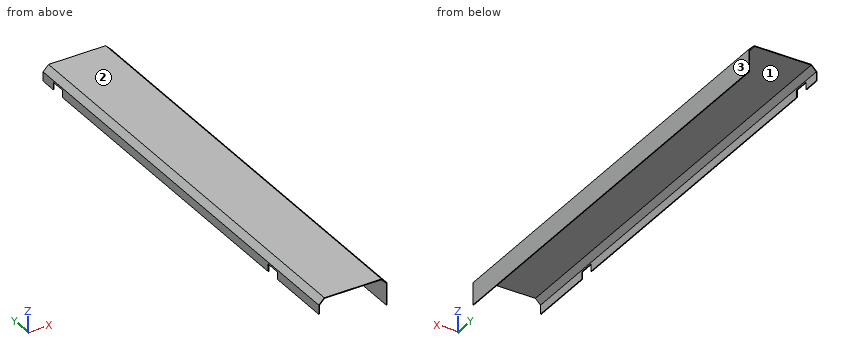
```python
from build123d import *

# Parameters (mm, degrees)
BOSS_EXTRUDE1_DEPTH = 1200
CUT_EXTRUDE1_REACH  = 187
SKETCH2_W           = 20
SKETCH2_H           = 40


with BuildPart() as part:
    # Sketch1 → Boss-Extrude1 (new body)
    with BuildSketch(Plane(origin=(0, 0, 0), x_dir=(1, 0, 0), z_dir=(0, 1, 0))):
        Polygon((15.828427125, 2), (2, 15.828427125), (2, 40), (0, 40), (0, 15), (15, 0), (170, 0), (185, 15), (185, 75), (183, 75), (183, 15.828427125), (169.171572875, 2), align=None)
    extrude(amount=BOSS_EXTRUDE1_DEPTH)

    # Sketch2 → Cut-Extrude1 (cut, up to next)
    with BuildSketch(Plane.ZY, mode=Mode.PRIVATE) as cut_extrude1_sk1:
        with Locations((-30, 200)):
            Rectangle(SKETCH2_W, SKETCH2_H)
    cut_extrude1_tool1 = extrude(cut_extrude1_sk1.sketch, amount=-CUT_EXTRUDE1_REACH, mode=Mode.PRIVATE) & part.part
    add(cut_extrude1_tool1.solids().sort_by_distance((0, 200, -30))[0], mode=Mode.SUBTRACT)
    # Sketch2 → Cut-Extrude1 (cut, up to next)
    with BuildSketch(Plane.ZY, mode=Mode.PRIVATE) as cut_extrude1_sk2:
        with Locations((-30, 1135)):
            Rectangle(SKETCH2_W, SKETCH2_H)
    cut_extrude1_tool2 = extrude(cut_extrude1_sk2.sketch, amount=-CUT_EXTRUDE1_REACH, mode=Mode.PRIVATE) & part.part
    add(cut_extrude1_tool2.solids().sort_by_distance((0, 1135, -30))[0], mode=Mode.SUBTRACT)


solid = part.part
```
Input: part model. Units: mm. Frame: model coordinates. Face numbers are marked on the shaded views. Give positions to 0.01 mm unless a question says otherwise; leave off trailing zeros. Order: outer loops, then holes, each group sorted by start corner. A loop starts at its lowest first (then second) coordinate and runs counter-clockwise, first axis right, second up. Notation, with made-up numbers: M 86.25,-21.75 L 142.25,-21.75 A17 cw 142.25,11.25 Z; hole C 66.5,66 d1. An arc over 180 degrees is marked long. Return JSON: item names as keys, results as strings.
1) Section query C-C on x = 100. Output: boundary loops of the cut face in (y, z), and give its area (3 significant figures).
Taken from the geometry:
{"outline": "M 0,-2 L 1200,-2 L 1200,0 L 0,0 Z", "area": "2,400 mm2"}
2) Mould query, pull axis X, two halves, no side actions, for the marked faces 1, 2 and 3. Classes: released by +X, released by -X, zero draft, split by the parting line, or undercut.
Taken from the geometry:
{"face 1": "undercut", "face 2": "zero draft", "face 3": "released by +X"}
3) Line query: L1, parallel to X at y = 661.5, z = -35; L2, parallel to Z at x = 65.5, y = 89.5; L3, parallel to X at y = 1005, z = -62. Output: solid intervals per line, ascending. Write a range as [from, to].
Taken from the geometry:
{"L1": "x = [0, 2], [183, 185]", "L2": "z = [-2, 0]", "L3": "x = [183, 185]"}
4) Section query A-A on y = 765.5. Output: boundary loops of the cut face in (x, z).
Taken from the geometry:
{"outline": "M 0,-40 L 2,-40 L 2,-15.83 L 15.83,-2 L 169.17,-2 L 183,-15.83 L 183,-75 L 185,-75 L 185,-15 L 170,0 L 15,0 L 0,-15 Z"}
5) Section query B-B on z = -53.5. Output: boundary loops of the cut face in (x, y), and give its area (3 significant figures).
Taken from the geometry:
{"outline": "M 183,0 L 185,0 L 185,1200 L 183,1200 Z", "area": "2,400 mm2"}
6) Contact query for flat-ended pins moving along their axis: pin 1 (1.6 mm diameter, centred on x = 1.5, y = 205, fed in from -Z); pin 2 (8 mm diameter, centred on x = 90.5, y = 407, fed in from +Z); pin 3 (1 mm diameter, centred on x = 1.5, y = 118, fed in from -Z); pin 4 (2 mm diameter, centred on x = 73, y = 730, fed in from -Z). Output: stop coordinate, or through.
Taken from the geometry:
{"pin 1": "stops at z = -20", "pin 2": "stops at z = 0", "pin 3": "stops at z = -40", "pin 4": "stops at z = -2"}
